CAD build for the part. Positions are in the model's coordinates, mm. A direction names the side the tool comes from. Coordinates: 2 decimals unless noted, no trailing zeros. Loops run counter-clockwise (first coordinate to the right, second up) from the corner with the lowest first, then second, coordinate; pieces in that order, holes last.
1) Two-plate mould, pull along X, no slides. Class faces 3 (the cylindrical face through (0.052, -26.037, -0.592)), 4 (the flat face through (9.35, 0, -0.4)), 5 (the cylindrical face through (9.85, 18.09, -0.61)), 6 (the flat face through (-9.8, 0, -0.5)): +X half, -X half, draft (parallel to the pull), parting line (faces both ways), or undercut.
2) Saw through at A-A, the plane x = 0. Write the cut outline in (y, z) (3 decimals), and give its area (3 significant figures).
3) Saw through at C-C, the plane z = -0.45. Write the cut outline in (x, y) (3 decimals).
4) Saw through at B-B, the plane y = 10.2. Write the cut outline in (x, z).
5) Which spindle directions (+Z, -Z, +X, -X, +Y, -Y) get a long thin tool onto all of the face, cutting with end or side? Do faces 1 (the flat face through (-9.35, -0.5, -0.4)), 2 (the flat face through (-10.15, 4, -1)). Say none if no direction does.
6) Wall check: line 1 along X through (y, z) = (10.2, -0.95); line 2 along X through (y, z) = (-13.5, -0.7); line 3 along Z through (x, y) = (-8, -12). Give the ranges that are in metal, low to high.
7) Pin check, flat tips, straight feed: pin 1 Ø0.5 at (y, z) = (0.5, -0.5) entering from -X; pin 2 Ø0.7 at (x, z) = (4, -0.5) entering from -Y; pin 3 Ø5 at (x, y) = (0, -14) entering from +Z. Stop position of each tip, or through.
8) Saw through at D-D, the plane y = -12. Write the cut outline in (x, z).
```python
from build123d import *

# Parameters (mm, degrees)
PAD011_DEPTH            = 2.2
SKETCH039_R             = 4
POCKET022_DEPTH         = 5
SKETCH040_R             = 2
POCKET027_DEPTH         = 5
POCKET023_DEPTH         = 0.85
SKETCH042_W             = 0.35
SKETCH042_H             = 0.6
POCKET024_DEPTH         = 25
FILLET004_R             = 1
SKETCH043_W             = 5
SKETCH043_H             = 1
POCKET029_DEPTH         = 0.35
SKETCH044_W             = 5
SKETCH044_H             = 1
POCKET028_DEPTH         = 0.35
BODY002_PLACEMENT_ANGLE = 180


with BuildPart() as part:
    # Sketch036 → Pad011 (new body)
    with BuildSketch(Plane.XY):
        with BuildLine():
            Line((-10.15, 18.375), (10.15, 18.375))
            Line((10.15, 18.375), (10.15, -17.75))
            Line((3.33, -24.57), (10.15, -17.75))
            ThreePointArc((-3.33, -24.57), (0, -26.037308), (3.33, -24.57))
            Line((-10.15, -17.75), (-3.33, -24.57))
            Line((-10.15, -17.75), (-10.15, 18.375))
        make_face()
    extrude(amount=PAD011_DEPTH)

    # Sketch039 → Pocket022 (cut)
    with BuildSketch(Plane.XY):
        with Locations((0, 10.2)):
            Circle(SKETCH039_R)
    extrude(amount=POCKET022_DEPTH, mode=Mode.SUBTRACT)

    # Sketch040 → Pocket027 (cut)
    with BuildSketch(Plane.XY):
        with Locations((0, -21.525)):
            Circle(SKETCH040_R)
    extrude(amount=POCKET027_DEPTH, mode=Mode.SUBTRACT)

    # Sketch041 → Pocket023 (cut)
    with BuildSketch(Plane.XY):
        with BuildLine():
            Line((-9.35, 17.285263), (-9.35, -17.814737))
            Line((-9.35, -17.814737), (-2.6, -24.564737))
            ThreePointArc((-2.6, -24.564737), (0, -25.525), (2.6, -24.564737))
            Line((2.6, -24.564737), (9.35, -17.814737))
            Line((9.35, -17.814737), (9.35, 17.285263))
            ThreePointArc((9.35, 17.285263), (9.155303, 17.755303), (8.685263, 17.95))
            Line((8.685263, 17.95), (-8.685263, 17.95))
            ThreePointArc((-8.685263, 17.95), (-9.155303, 17.755303), (-9.35, 17.285263))
        make_face()
    extrude(amount=POCKET023_DEPTH, mode=Mode.SUBTRACT)

    # Sketch042 (on Face16 of Pocket023) → Pocket024 (cut)
    with BuildSketch(Plane.YZ.offset(-9.35)):
        with Locations((-9.625, -1.8)):
            Rectangle(SKETCH042_W, SKETCH042_H)
        with Locations((9.625, -1.8)):
            Rectangle(SKETCH042_W, SKETCH042_H)
    extrude(amount=-POCKET024_DEPTH, mode=Mode.SUBTRACT)

    # Fillet004
    fillet004_edges = [part.edges().sort_by_distance(p)[0] for p in [
        (10.15, -17.75, 1.1),
        (10.15, 18.375, 1.1),
        (-6.74, -21.16, 2.2),
        (-10.15, 0.3125, 2.2),
        (0, -26.037308, 2.2),
        (0, 18.375, 2.2),
        (6.74, -21.16, 2.2),
        (10.15, 0.3125, 2.2),
        (-2, -21.525, 2.2),
        (-4, 10.2, 2.2),
        (-10.15, 18.375, 1.1),
        (-10.15, -17.75, 1.1),
    ]]
    fillet(fillet004_edges, radius=FILLET004_R)

    # Sketch043 (on Face10 of Fillet004) → Pocket029 (cut)
    with BuildSketch(Plane(origin=(-10.15, 0, 0), x_dir=(0, -1, 0), z_dir=(-1, 0, 0))):
        with Locations((0, 0.5)):
            Rectangle(SKETCH043_W, SKETCH043_H)
    extrude(amount=-POCKET029_DEPTH, mode=Mode.SUBTRACT)

    # Sketch044 (on Face11 of Pocket029) → Pocket028 (cut)
    with BuildSketch(Plane.YZ.offset(10.15)):
        with Locations((0, 0.5)):
            Rectangle(SKETCH044_W, SKETCH044_H)
    extrude(amount=-POCKET028_DEPTH, mode=Mode.SUBTRACT)


with BuildPart() as part_1:
    # Body002 placement: moved
    add(part.part.rotate(Axis((0, 0, 0), (0, 1, 0)), BODY002_PLACEMENT_ANGLE))


solid = part_1.part
```
Data:
1. face 3: parting line
1. face 4: undercut
1. face 5: +X half
1. face 6: -X half
2. outline: (-26.037, -1.2) arc R1 ccw to (-25.037, -2.2) - (-24.525, -2.2) arc R1 ccw to (-23.525, -1.2) - (-23.525, -0.85) - (-25.525, -0.85) - (-25.525, 0) - (-26.037, 0) - close; (-19.525, -1.2) arc R1 ccw to (-18.525, -2.2) - (5.2, -2.2) arc R1 ccw to (6.2, -1.2) - (6.2, -0.85) - (-19.525, -0.85) - close; (14.2, -1.2) arc R1 ccw to (15.2, -2.2) - (17.375, -2.2) arc R1 ccw to (18.375, -1.2) - (18.375, 0) - (17.95, 0) - (17.95, -0.85) - (14.2, -0.85) - close
2. area: 43.3 mm2
3. outline: (-10.15, -17.336) arc R1 ccw to (-9.857, -18.043) - (-3.33, -24.57) arc R4.512 ccw to (3.33, -24.57) - (9.857, -18.043) arc R1 ccw to (10.15, -17.336) - (10.15, -2.5) - (9.8, -2.5) - (9.8, 2.5) - (10.15, 2.5) - (10.15, 17.375) arc R1 ccw to (9.15, 18.375) - (-9.15, 18.375) arc R1 ccw to (-10.15, 17.375) - (-10.15, 2.5) - (-9.8, 2.5) - (-9.8, -2.5) - (-10.15, -2.5) - close; hole (-9.35, -17.815) - (-2.6, -24.565) arc R4 ccw to (2.6, -24.565) - (9.35, -17.815) - (9.35, 17.285) arc R0.665 ccw to (8.685, 17.95) - (-8.685, 17.95) arc R0.665 ccw to (-9.35, 17.285) - close
4. outline: (-10.15, -1.2) arc R1 ccw to (-9.15, -2.2) - (-5, -2.2) arc R1 ccw to (-4, -1.2) - (-4, -0.85) - (-9.35, -0.85) - (-9.35, 0) - (-10.15, 0) - close; (4, -1.2) arc R1 ccw to (5, -2.2) - (9.15, -2.2) arc R1 ccw to (10.15, -1.2) - (10.15, 0) - (9.35, 0) - (9.35, -0.85) - (4, -0.85) - close
5. face 1: +Z
5. face 2: +Z, -Z, -X, +Y, -Y
6. line 1: x = -10.15 to -4, 4 to 10.15
6. line 2: x = -10.15 to -9.35, 9.35 to 10.15
6. line 3: z = -2.2 to -0.85
7. pin 1: stops at x = -9.8
7. pin 2: stops at y = -24.25
7. pin 3: stops at z = -0.85
8. outline: (-10.15, -1.2) arc R1 ccw to (-9.15, -2.2) - (9.15, -2.2) arc R1 ccw to (10.15, -1.2) - (10.15, 0) - (9.35, 0) - (9.35, -0.85) - (-9.35, -0.85) - (-9.35, 0) - (-10.15, 0) - close
